Design review of the part built by this model. Coordinates are the model's own, in mm. A direction names the side the tool comes from. Coordinates: 2 decimals unless noted, no trailing zeros. Write each loop counter-clockwise with the first axis right and the second up, starting at its lowest first coordinate (ties: lowest second). Pieces come first, ordered by that corner, then holes. Notation, with made-up numbers: M -8,8 L 23,8 A34 cw 23,42 Z; hole C -35,-16.75 d3. An arc over 180 degrees is marked long. One line per question, with ' | ' between items.
Autodesk Inventor part; units mm, degrees
ref_plane "YZ Plane" through (0, 0, 0) normal (1, 0, 0) x (0, 1, 0)
ref_plane "XZ Plane" through (0, 0, 0) normal (0, 1, 0) x (-1, 0, 0)
ref_plane "XY Plane" through (0, 0, 0) normal (0, 0, 1) x (1, 0, 0)
sketch "スケッチ1" plane through (0, 0, 0) normal (0, 0, 1) x (1, 0, 0)
  line L0 (18.3733, -7.7435) -> (14.2723, -7.7348)
  arc A0 (18.3733, -7.7435) -> (20.0717, -6.1303) centre (18.4564, -6.1303) ccw
  line L1 (20.0717, -2.0205) -> (20.0717, -6.1303)
  line L2 (18.408, 0) -> (-1.0303, 0)
  arc A1 (-1.0303, 0) -> (-2.9281, -1.8978) centre (-1.0303, -1.8978) ccw
  line L3 (-2.9281, -1.8978) -> (-2.9281, -6.5862)
  arc A2 (-2.9281, -6.5862) -> (-0.7099, -8.8044) centre (-0.7099, -6.5862) ccw
  arc A3 (26.8795, -33.0792) -> (27.974, -33.1771) centre (27.7186, -29.8656) ccw
  line L4 (29.6865, -31.7299) -> (27.974, -33.1771)
  arc A4 (29.6865, -31.7299) -> (31.4665, -28.292) centre (32.5726, -31.0444) ccw
  line L5 (31.4665, -28.292) -> (14.2723, -7.7348)
  circle A5 centre (16.0858, -4.066) radius 2.5
  line L6 (4.5899, -0.941) -> (1.1333, -0.941)
  arc A6 (4.3798, -7.1842) -> (4.5899, -0.941) centre (4.5858, -4.066) ccw
  line L7 (4.3798, -7.1842) -> (1.0695, -7.1903)
  arc A7 (1.1333, -0.941) -> (1.0695, -7.1903) centre (1.1379, -4.066) ccw
  line L8 (26.8795, -33.0792) -> (6.576, -8.8044)
  line L9 (-0.7099, -8.8044) -> (6.576, -8.8044)
  arc A8 (20.0717, -2.0205) -> (18.408, 0) centre (18.013, -2.0205) ccw
  point P0 (0, 0)
  dimension "d0" = 5
  dimension "d1" = 3.125
  dimension "d17" = 4.8539
  dimension "d24" = 11.5
  dimension "d29" = 14.9479
  dimension "d44" = 4.066
  dimension "d45" = 4.066
  dimension "d46" = 90
  dimension "d47" = 90
  dimension "d48" = 3.125
extrude "押し出し1" add sketch "スケッチ1" along normal blind 10.6
sketch "スケッチ2" plane through (0, 0, 10.6) normal (0, 0, 1) x (1, 0, 0)
  point P0 (0, 0)
sketch "スケッチ3" plane through (0, 0, 10.6) normal (0, 0, 1) x (1, 0, 0)
  arc A0 (29.6865, -31.7299) -> (31.4665, -28.292) centre (32.5726, -31.0444) ccw
  arc A1 (31.4665, -28.292) -> (29.6865, -31.7299) centre (32.5726, -31.0444) ccw
  point P0 (0, 0)
extrude "押し出し2" add sketch "スケッチ3" along normal blind 20
equation "\"d45\" = d44"
equation "\"d48\" = d1"
1. Take a section at B-B (x = 5.5). Write out the cut boundary in (y, z).
Answer sheet:
outline: M -8.8,0 L -7.05,0 L -7.05,10.6 L -8.8,10.6 Z; M -1.08,0 L 0,0 L 0,10.6 L -1.08,10.6 Z
2. Take a section at A-A (x = 17). Write out the cut boundary in (y, z), then the cut area to 3 significant figures.
Answer sheet:
outline: M -21.27,0 L -11,0 L -11,10.6 L -21.27,10.6 Z; M -7.74,0 L -6.39,0 L -6.39,10.6 L -7.74,10.6 Z; M -1.74,0 L 0,0 L 0,10.6 L -1.74,10.6 Z | area: 142 mm^2
3. Draft analysis for pull direction Y (two halves, no side actions). For faces 4 (the face through (22.99, -18.16, 5.23)), 5 (the face through (15, -14, 10.6)), 6 (the face through (-2.387, -0.571, 5.226)), state which applies: pulls with the +Y half, pulls with the -Y half, needs draft (parallel to the pull), parting line crosses it, or undercut.
Answer sheet:
face 4: undercut | face 5: needs draft | face 6: pulls with the +Y half
4. Tool access review of faces 1 (the face through (29.925, -29.707, 20.46)), 2 (the face through (28.842, -32.443, 5.226)), 3 (the face through (-2.261, -8.172, 5.226)): name each direction out of +Z, -Z, +X, -X, +Y, -Y from which nothing blocks a thin tool from reaching the whole face with its end or side.
Answer sheet:
face 1: +Z, -X | face 2: +Z, -Z, -Y | face 3: +Z, -Z, -X, -Y
5. To check wall thickness, follow line 1 along Z through (x, y) = (19.5, -18.5); line 2 along Y through (x, z) = (2.5, 6.5); line 3 along X through (y, z) = (-21, 3.5). State the ranges of each line that lie inside material, in increasing order. Write a range as [from, to].
Answer sheet:
line 1: [0, 10.6] | line 2: [-8.8, -7.19], [-0.94, 0] | line 3: [16.78, 25.37]
6. Take a section at D-D (z = 7.5). Count the separate pieces of the cut face and the enclosed holes in it, then the cut area to 3 significant figures.
Answer sheet:
separate pieces: 1 | enclosed holes: 2 | area: 340 mm^2
7. Take a section at C-C (z = 22). Write out the cut boundary in (x, y), then the cut area to 3 significant figures.
Answer sheet:
outline: M 29.69,-31.73 A2.97 ccw long 31.47,-28.29 A2.97 ccw Z | area: 27.6 mm^2
8. Insertion check: pin 1 Ø3 at (x, y) = (14, -21) entering from -Z; pin 2 Ø8 at (x, z) = (1.5, 4) entering from -Y; pin 3 Ø1.2 at (y, z) = (-5, 3.5) entering from +X; pin 4 Ø5 at (x, y) = (23.5, -17.5) entering from +Z. Each pin has a flat end and moves straight along its axis. Give the tip position at first contact, or say it passes through.
Answer sheet:
pin 1: through | pin 2: y = -8.8 | pin 3: x = 20.07 | pin 4: z = 10.6
